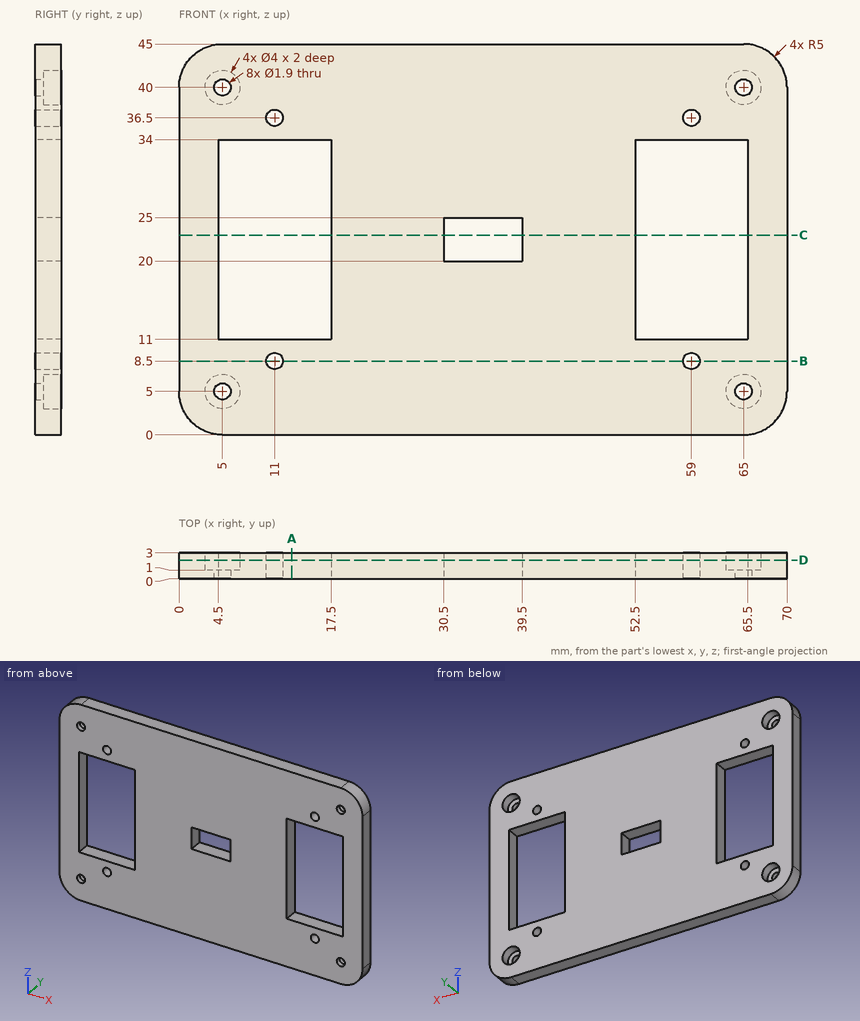
Check sheet for the drawn part. Datum: minimum x, y, z corner. Units: mm. Give positions to 0.01 mm unless a question says otherwise; leave off trailing zeros. Order: outer loops, then holes, each group sorted by start corner. A loop starts at its lowest first (then second) coordinate and runs counter-clockwise, first axis right, second up. Notation, with made-up numbers: (37.5, 2.5) -> (89.5, 2.5) arc R18 ccw to (89.5, 6.5) -> close; hole circle Ø8 at (25.5, 84). An arc over 180 degrees is marked (long way). One line per item, written item: value.
(1) Sectioned sample at B-B on z = 8.5. Record the cut outline in (x, y).
Final values:
outline: (0, 0) -> (10.05, 0) -> (10.05, 3) -> (0, 3) -> close; (11.95, 0) -> (58.05, 0) -> (58.05, 3) -> (11.95, 3) -> close; (59.95, 0) -> (70, 0) -> (70, 3) -> (59.95, 3) -> close
(2) Sectioned sample at A-A on x = 13. Record the cut outline in (y, z), then the cut area to 3 significant figures.
Final values:
outline: (0, 0) -> (3, 0) -> (3, 11) -> (0, 11) -> close; (0, 34) -> (3, 34) -> (3, 45) -> (0, 45) -> close
area: 66.0 mm^2
(3) Scan lines: line 1 along X through (y, z) = (1, 27); line 2 along X through (y, z) = (2, 5); line 3 along Z through (x, y) = (65, 2.1). Record each from-to range of solid material in increasing order. Write a range as [from, to].
Final values:
line 1: [0, 4.5], [17.5, 52.5], [65.5, 70]
line 2: [0, 3], [7, 63], [67, 70]
line 3: [0, 3], [7, 11], [34, 38], [42, 45]
(4) Gauge pin test, flat end, axial feed: pin 1 (1.2 mm diameter, centred on x = 4.5, z = 5.5, fed in from +Y). Record the tip position at first contact, or that the pin passes through.
Final values:
pin 1: y = 1
(5) Sectioned sample at C-C on z = 23. Record the cut outline in (x, y), then the cut area to 3 significant figures.
Final values:
outline: (0, 0) -> (4.5, 0) -> (4.5, 3) -> (0, 3) -> close; (17.5, 0) -> (30.5, 0) -> (30.5, 3) -> (17.5, 3) -> close; (39.5, 0) -> (52.5, 0) -> (52.5, 3) -> (39.5, 3) -> close; (65.5, 0) -> (70, 0) -> (70, 3) -> (65.5, 3) -> close
area: 105 mm^2
(6) Sectioned sample at D-D on y = 2.15. Count the separate pieces of the cut face and the enclosed holes in it, then the cut area to 3 significant figures.
Final values:
separate pieces: 1
enclosed holes: 11
area: 2,420 mm^2
